Answer from the drawing. Dimensions are ordinates in mm from the lowest x, y and z of the part. A direction names the side the tool comes from. Round coordinates to 2 decimals unless told otherwise and drop trailing zeros. Order: outer loops, then holes, each group sorted by start corner. A loop starts at its lowest first (then second) coordinate and runs counter-clockwise, first axis right, second up. Notation, with made-up numbers: (39.5, -38.5) - (55.5, -38.5) arc R30 cw to (55.5, -3.5) - close; hole circle Ø1 at (-29.75, -27). An arc over 180 degrees is marked (long way). One line per question, with ' | ' between items. Start each with the question number.
1) The part is cut by section B-B, the plane z = 4.75. Give the vertices of the cut face in (x, y), plus the area to 3 significant figures.
2) The mould has two halves that part along X. Classify the marked faces 1, 2, 3 and 4: pulls with the +X half, pulls with the -X half, needs draft (parallel to the pull), parting line crosses it, or undercut.
3) The part is cut by section D-D, the plane y = 9. Give the vertices of the cut face in (x, z), plus the area to 3 significant figures.
4) For the marked faces 5, 6 and 7, determine the directions among +Z, -Z, +X, -X, +Y, -Y from which every point of the face is accessible in a straight line to the end or side of a thin tool.
5) The part is cut by section A-A, the plane y = 5. Give the vertices of the cut face in (x, z), plus the area to 3 significant figures.
6) The part is cut by section C-C, the plane x = 12. Give the vertices of the cut face in (y, z).
7) Flat-ended cylindrical pins translate along their axes: pin 1 (1.8 mm diameter, centred on x = 12, y = 5, fed in from +Z); pin 2 (3 mm diameter, centred on x = 12.5, y = 6, fed in from +Z); pin 3 (1.3 mm diameter, centred on y = 7, z = 6, fed in from -X); pin 4 (2 mm diameter, centred on y = 4.5, z = 6, fed in from +X). Find the tip coordinate at first contact, or state that the pin passes through.
8) Straight lines are drawn through the part: line 1 (X direction, y = 7.25, z = 5.25); line 2 (Y direction, x = 12, z = 1.45); line 3 (X direction, y = 5, z = 0.85). For each, find the intervals that lie inside material, in ascending order. Write a range as from..to.
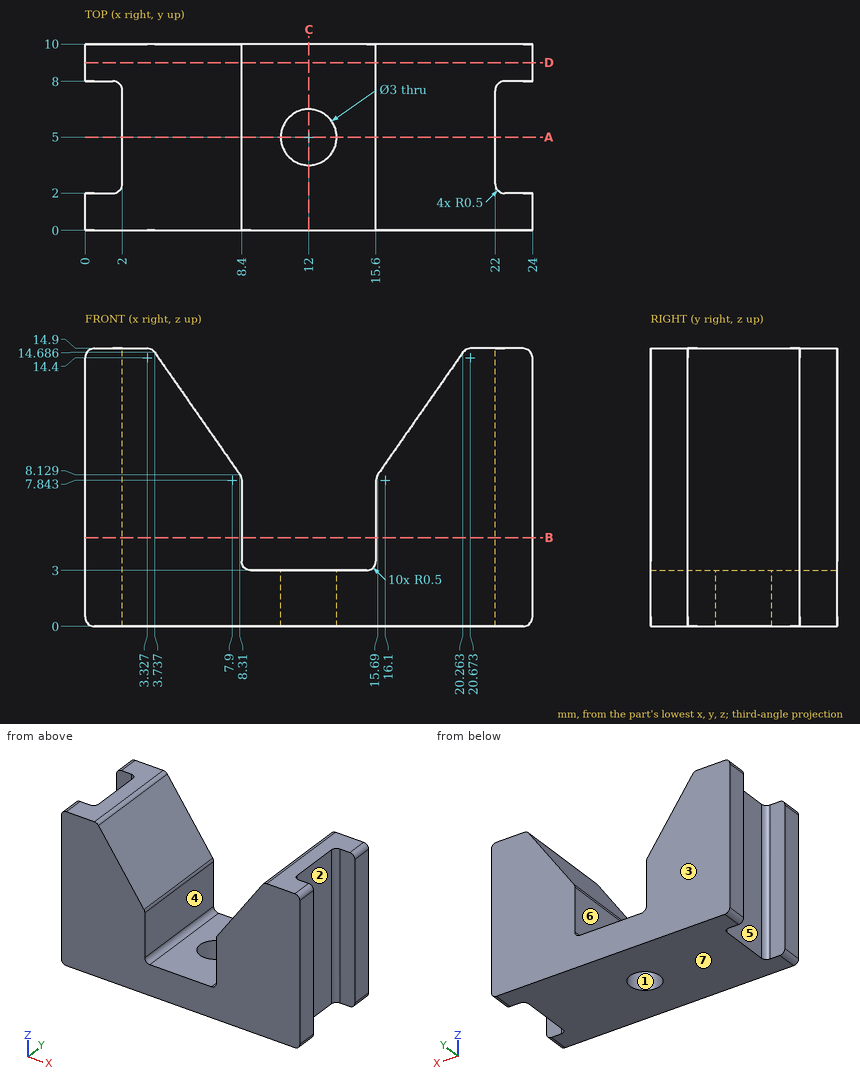
Values:
1) outline: (0, 0) - (8.4, 0) - (8.4, 10) - (0, 10) - (0, 8) - (1.5, 8) arc R0.5 cw to (2, 7.5) - (2, 2.5) arc R0.5 cw to (1.5, 2) - (0, 2) - close; (15.6, 0) - (24, 0) - (24, 2) - (22.5, 2) arc R0.5 cw to (22, 2.5) - (22, 7.5) arc R0.5 cw to (22.5, 8) - (24, 8) - (24, 10) - (15.6, 10) - close | area: 144 mm^2
2) face 1: undercut | face 2: pulls with the +X half | face 3: needs draft | face 4: undercut
3) outline: (0, 0.5) arc R0.5 ccw to (0.5, 0) - (23.5, 0) arc R0.5 ccw to (24, 0.5) - (24, 14.4) arc R0.5 ccw to (23.5, 14.9) - (20.67, 14.9) arc R0.5 ccw to (20.26, 14.69) - (15.69, 8.13) arc R0.5 ccw to (15.6, 7.84) - (15.6, 3.5) arc R0.5 cw to (15.1, 3) - (8.9, 3) arc R0.5 cw to (8.4, 3.5) - (8.4, 7.84) arc R0.5 ccw to (8.31, 8.13) - (3.74, 14.69) arc R0.5 ccw to (3.33, 14.9) - (0.5, 14.9) arc R0.5 ccw to (0, 14.4) - close | area: 239 mm^2
4) face 5: +Z, -Z, -X | face 6: +Z, +Y, -Y | face 7: -Z, +X, -X, +Y, -Y
5) outline: (2, 0) - (10.5, 0) - (10.5, 3) - (8.9, 3) arc R0.5 cw to (8.4, 3.5) - (8.4, 7.84) arc R0.5 ccw to (8.31, 8.13) - (3.74, 14.69) arc R0.5 ccw to (3.33, 14.9) - (2, 14.9) - close; (13.5, 0) - (22, 0) - (22, 14.9) - (20.67, 14.9) arc R0.5 ccw to (20.26, 14.69) - (15.69, 8.13) arc R0.5 ccw to (15.6, 7.84) - (15.6, 3.5) arc R0.5 cw to (15.1, 3) - (13.5, 3) - close | area: 170 mm^2
6) outline: (0, 0) - (3.5, 0) - (3.5, 3) - (0, 3) - close; (6.5, 0) - (10, 0) - (10, 3) - (6.5, 3) - close
7) pin 1: passes through | pin 2: stops at z = 3 | pin 3: stops at x = 1.98 | pin 4: stops at x = 22
8) line 1: x = 2..8.4, 15.6..22 | line 2: y = 0..3.5, 6.5..10 | line 3: x = 2..10.5, 13.5..22
